Check sheet for the modelled part. Datum: model origin and axes. Units: mm. Coordinates: 2 decimals unless noted, no trailing zeros. Loops run counter-clockwise (first coordinate to the right, second up) from the corner with the lowest first, then second, coordinate; pieces in that order, holes last. Notation, with made-up numbers: (12, -5) - (18, -5) arc R14 cw to (18, 1) - close; hole circle Ø8 at (26.5, -1.75). An arc over 180 degrees is marked (long way). Write each question's results on one line, items separated by ' | '. Start each with the question number.
1. Cross-section at D-D (y = -7.5). Record the cut outline in (x, z) (1 decimal), and give its area (3 significant figures).
2. Draft check along Y on faces 1 (the face through (77.88, -10.74, 2.38)), 2 (the face through (8.414, -8.358, -0.07)), 3 (the face through (77.88, -2.3, -5.54)). Enter one of: released by +Y, released by -Y, zero draft, split by the parting line, or undercut.
3. Thickness scan on line 1 (X direction, y = 8.3, z = 0) (1 decimal); line 2 (Y direction, x = 141, z = 0.5); line 3 (Z direction, x = 10, y = -9.2). Record the ranges inside material, lowest first. Write a range as [from, to].
4. Cross-section at A-A (y = 0). Record the cut outline in (x, z) (3 decimals), and give its area (3 significant figures).
5. Gauge pin test, flat ends, axial feed: P1, Ø5, axis at x = 56.5, z = 3.5, coming from the -Y side; P2, Ø4, axis at x = 93, z = 5.5, coming from the -Y side; P3, Ø1.5, axis at x = 114.5, y = -5.5, coming from the -Z side. Record the tip position at first contact, or that the pin passes through.
6. Cross-section at C-C (x = 10). Record the cut outline in (y, z).
7. Cross-section at B-B (z = 0). Record the cut outline in (x, y) (1 decimal).
```python
from build123d import *

# Parameters (mm, degrees)
SKETCH2_R               = 11
SKETCH2_R_2             = 6
BOSS_EXTRUDE1_DEPTH     = 157.975
SKETCH3_R               = 1.5875
CUT_EXTRUDE1_DEPTH      = 12
CUT_EXTRUDE1_DEPTH_BACK = 12


with BuildPart() as part:
    # Sketch2 → Boss-Extrude1 (new body)
    with BuildSketch(Plane(origin=(0, 0, 0), x_dir=(0, 0, -1), z_dir=(1, 0, 0))):
        Circle(SKETCH2_R)
        Circle(SKETCH2_R_2, mode=Mode.SUBTRACT)
    extrude(amount=BOSS_EXTRUDE1_DEPTH)

    # Sketch3 → Cut-Extrude1 (cut, two sides)
    with BuildSketch(Plane(origin=(0, 0, 0), x_dir=(1, 0, 0), z_dir=(0, 1, 0))) as cut_extrude1_sk:
        with Locations((10, 0)):
            Circle(SKETCH3_R)
        with Locations((147.975, 0)):
            Circle(SKETCH3_R)
    extrude(amount=CUT_EXTRUDE1_DEPTH, mode=Mode.SUBTRACT)
    extrude(cut_extrude1_sk.sketch, amount=-CUT_EXTRUDE1_DEPTH_BACK, mode=Mode.SUBTRACT)


solid = part.part
```
Established:
1) outline: (0, -8) - (158, -8) - (158, 8) - (0, 8) - close; hole circle Ø3.2 at (10, 0); hole circle Ø3.2 at (148, 0) | area: 2,530 mm^2
2) face 1: split by the parting line | face 2: zero draft | face 3: undercut
3) line 1: [0, 8.4], [11.6, 146.4], [149.6, 158] | line 2: [-10.99, -5.98], [5.98, 10.99] | line 3: [-6.03, -1.59], [1.59, 6.03]
4) outline: (0, -11) - (157.975, -11) - (157.975, -6) - (0, -6) - close; (0, 6) - (157.975, 6) - (157.975, 11) - (0, 11) - close | area: 1,580 mm^2
5) P1: y = -10.95 | P2: y = -10.43 | P3: z = -9.92
6) outline: (-10.88, -1.59) arc R11 ccw to (10.88, -1.59) - (5.79, -1.59) arc R6 cw to (-5.79, -1.59) - close; (-10.88, 1.59) - (-5.79, 1.59) arc R6 cw to (5.79, 1.59) - (10.88, 1.59) arc R11 ccw to start
7) outline: (0, -11) - (8.4, -11) - (8.4, -6) - (0, -6) - close; (0, 6) - (8.4, 6) - (8.4, 11) - (0, 11) - close; (11.6, -11) - (146.4, -11) - (146.4, -6) - (11.6, -6) - close; (11.6, 6) - (146.4, 6) - (146.4, 11) - (11.6, 11) - close; (149.6, -11) - (158, -11) - (158, -6) - (149.6, -6) - close; (149.6, 6) - (158, 6) - (158, 11) - (149.6, 11) - close
